The model under review builds one solid part; all positions refer to its coordinate system, in mm. A direction names the side the tool comes from. Round coordinates to 2 decimals unless told otherwise and drop trailing zeros. Write each loop counter-clockwise with the first axis right and the second up, starting at its lowest first coordinate (ties: lowest second). Pieces come first, ordered by that corner, then holes. Notation, with made-up numbers: (32, 60) -> (79, 60) arc R33 ccw to (79, 91) -> close; hole circle Ø7 at (24.25, 25). An arc over 180 degrees is marked (long way). Answer as a JSON object with one key per item and string values. Group by question number.
1) Machinability: for faces 1 (the flat face through (0, 4.5, 12)), 2 (the flat face through (0, 5, 8.7)), 3 (the flat face through (9.2, -3.4, 8.7)), which of the approach directions +Z, -Z, +X, -X, +Y, -Y give a long, thin tool a straight path to every point of the face, cutting with its end or side? Answer none if there is none.
2) We need section A-A, the plane y = -2.5. Write out the cut boundary in (x, z), then the cut area to 3 significant figures.
3) Insertion check: pin 1 Ø1.5 at (x, y) = (2, -6.5) entering from -Z; pin 2 Ø1 at (x, z) = (6.5, 30.5) entering from +Y; pin 3 Ø4 at (y, z) = (-5, 12) entering from +X. Each pin has a flat end and moves straight along its axis. Give the tip position at first contact, or say it passes through.
4) We need section B-B, the plane z = 20.5. Write out the cut boundary in (x, y).
5) We need section C-C, the plane x = -8. Write out the cut boundary in (y, z), then the cut area to 3 significant figures.
6) To check wall thickness, follow probe 1 along X at (y, z) = (1.75, 32); probe 2 along Y at (x, z) = (4, 2.5); probe 3 along Z at (x, y) = (3.25, -6.25). State the ranges of each line that lie inside material, in increasing order. Write a range as [from, to].
7) We need section D-D, the plane y = 2.5. Write out the cut boundary in (x, z).
from build123d import *

# Parameters (mm, degrees)
EXTRUDE_1_DEPTH  = 8.7
EXTRUDE_2_DEPTH  = 6
EXTRUDE_7_DEPTH  = 22
EXTRUDE_15_REACH = 42.002
SKETCH_6_W       = 12.4
SKETCH_6_H       = 36.7
EXTRUDE_16_REACH = 46.194
SKETCH_10_W      = 12
SKETCH_10_H      = 1
SKETCH_11_W      = 12.4
SKETCH_11_H      = 22
EXTRUDE_17_DEPTH = 3


with BuildPart() as part:
    # ｽｹｯﾁ1 → ﾎﾞｽ - 押し出し1 (new body)
    with BuildSketch(Plane.XY):
        with BuildLine():
            Line((-6, 5.5), (6, 5.5))
            ThreePointArc((6, 5.5), (11.5, 0), (6, -5.5))
            Line((6, -5.5), (-6, -5.5))
            ThreePointArc((-6, -5.5), (-11.5, 0), (-6, 5.5))
        make_face()
    extrude(amount=EXTRUDE_1_DEPTH)

    # ｽｹｯﾁ4 → ﾎﾞｽ - 押し出し2 (add)
    with BuildSketch(Plane.XY.offset(8.7)):
        with BuildLine():
            Line((-6, -4.5), (6, -4.5))
            ThreePointArc((6, -4.5), (10.5, 0), (6, 4.5))
            Line((6, 4.5), (-6, 4.5))
            ThreePointArc((-6, 4.5), (-10.5, 0), (-6, -4.5))
        make_face()
    extrude(amount=EXTRUDE_2_DEPTH)

    # ｽｹｯﾁ5 → ﾎﾞｽ - 押し出し7 (add)
    with BuildSketch(Plane.XY.offset(14.7)):
        with BuildLine():
            ThreePointArc((-3.45, 1.02834819), (-10.5, 0), (-3.45, -1.02834819))
            ThreePointArc((-3.45, -1.02834819), (0, -3.6), (3.45, -1.02834819))
            ThreePointArc((3.45, -1.02834819), (10.5, 0), (3.45, 1.02834819))
            ThreePointArc((3.45, 1.02834819), (0, 3.6), (-3.45, 1.02834819))
        make_face()
    extrude(amount=EXTRUDE_7_DEPTH)

    # ｽｹｯﾁ6 → ﾎﾞｽ - 押し出し15 (add, up to next)
    with BuildSketch(Plane.XZ.offset(5.5), mode=Mode.PRIVATE) as extrude_15_sk1:
        with Locations((0, 18.35)):
            Rectangle(SKETCH_6_W, SKETCH_6_H)
    extrude_15_tool1 = extrude(extrude_15_sk1.sketch, amount=-EXTRUDE_15_REACH, mode=Mode.PRIVATE) - part.part
    add(extrude_15_tool1.solids().sort_by_distance((0, -5.5, 18.35))[0])

    # ｽｹｯﾁ10 → ﾎﾞｽ - 押し出し16 (add, up to next)
    with BuildSketch(Plane(origin=(12.5, 0, 0), x_dir=(0, 0, -1), z_dir=(1, 0, 0)), mode=Mode.PRIVATE) as extrude_16_sk1:
        with Locations((-6, 0)):
            Rectangle(SKETCH_10_W, SKETCH_10_H)
    extrude_16_tool1 = extrude(extrude_16_sk1.sketch, amount=-EXTRUDE_16_REACH, mode=Mode.PRIVATE) - part.part
    extrude_16 = extrude_16_tool1.solids().sort_by_distance((12.5, 0, 6))[0]
    add(extrude_16)

    # ﾐﾗｰ1: ﾎﾞｽ - 押し出し16 across plane
    add(extrude_16.mirror(Plane(origin=(0, 0, 0), x_dir=(0, 0, 1), z_dir=(1, 0, 0))))

    # ｽｹｯﾁ11 → ﾎﾞｽ - 押し出し17 (add)
    with BuildSketch(Plane.XZ.offset(5.5)):
        with Locations((0, 25.7)):
            Rectangle(SKETCH_11_W, SKETCH_11_H)
    extrude(amount=EXTRUDE_17_DEPTH)


solid = part.part
Here are the results:
{
 "1": {"face 1": "+Z, +X, -X, +Y", "face 2": "+Z, +Y", "face 3": "+Z, +X, -Y"},
 "2": {"outline": "(-10.9, 0) -> (10.9, 0) -> (10.9, 8.7) -> (9.74, 8.7) -> (9.74, 14.7) -> (9.49, 14.7) -> (9.49, 36.7) -> (-9.49, 36.7) -> (-9.49, 14.7) -> (-9.74, 14.7) -> (-9.74, 8.7) -> (-10.9, 8.7) -> close", "area": "724 mm^2"},
 "3": {"pin 1": "stops at z = 14.7", "pin 2": "stops at y = 3.6", "pin 3": "stops at x = 9.35"},
 "4": {"outline": "(-6.2, -8.5) -> (6.2, -8.5) -> (6.2, -3.53) arc R3.6 ccw (long way) to (3.45, 1.03) arc R3.6 ccw to (-3.45, 1.03) arc R3.6 ccw (long way) to (-6.2, -3.53) -> close"},
 "5": {"outline": "(-5.12, 0) -> (5.12, 0) -> (5.12, 8.7) -> (4.03, 8.7) -> (4.03, 14.7) -> (3.43, 14.7) -> (3.43, 36.7) -> (-3.43, 36.7) -> (-3.43, 14.7) -> (-4.03, 14.7) -> (-4.03, 8.7) -> (-5.12, 8.7) -> close", "area": "288 mm^2"},
 "6": {"probe 1": "x = [-10.05, -3.75], [-3.15, 3.15], [3.75, 10.05]", "probe 2": "y = [-5.5, 5.5]", "probe 3": "z = [14.7, 36.7]"},
 "7": {"outline": "(-10.9, 0) -> (10.9, 0) -> (10.9, 8.7) -> (9.74, 8.7) -> (9.74, 14.7) -> (9.49, 14.7) -> (9.49, 36.7) -> (4.31, 36.7) -> (4.31, 14.7) -> (2.59, 14.7) -> (2.59, 36.7) -> (-2.59, 36.7) -> (-2.59, 14.7) -> (-4.31, 14.7) -> (-4.31, 36.7) -> (-9.49, 36.7) -> (-9.49, 14.7) -> (-9.74, 14.7) -> (-9.74, 8.7) -> (-10.9, 8.7) -> close"}
}
